Model file for the job. Use its own axes, mm. Face numbers are marked on the shaded views. A direction names the side the tool comes from. Give positions to 0.01 mm unless a question says otherwise; leave off trailing zeros. Loops run counter-clockwise (first coordinate to the right, second up) from the corner with the lowest first, then second, coordinate; pieces in that order, holes last. Notation, with made-up numbers: (12.25, 49.25) -> (61.25, 49.25) arc R31 cw to (61.25, 77.25) -> close; hole circle Ø10 at (31, -14.75). An arc over 180 degrees is marked (long way). Use CSV: the item, a comma, the result in double quotes. Start each with the question number.
(1) Drill centre lines: probe 1 along X at (y, z) = (143.5, 17); probe 2 along X at (y, z) = (-10, 54.5); probe 3 along Z at (x, y) = (19.5, -4). Where is each one in solid material? Low to high.
(2) Cut at A-A on z = -134. Write the cut outline in (x, y).
(3) Cut at D-D on x = 14. Write the cut outline in (y, z).
(4) 3-axis set-ups, long thin cutter, end or side, ignore diameter. For the marked faces 3, 4, 5 and 6: which of +Z, -Z, +X, -X, +Y, -Y reach the whole face in a straight line?
(5) Cut at B-B on x = -82. Write the cut outline in (y, z), then the cut area to 3 significant figures.
(6) Pull direction Y, two halves, no side cores. Call the marked faces 1 and 2: pulls with the +Y half, pulls with the -Y half, needs draft (parallel to the pull), parting line crosses it, or undercut.
(7) Flat gauge pins, fed straight in: pin 1 (5 mm diameter, centred on x = -75, z = -80, fed in from +Y); pin 2 (1 mm diameter, centred on x = 175, y = -15.5, fed in from +Z); pin 3 (10 mm diameter, centred on x = -44.5, z = 64.5, fed in from -Y); pin 4 (7.5 mm diameter, centred on y = -35.27, z = -48.54, fed in from +X). Where does each tip first touch, or does it go through?
(8) Cut at C-C on y = 127. Write the cut outline in (x, z).
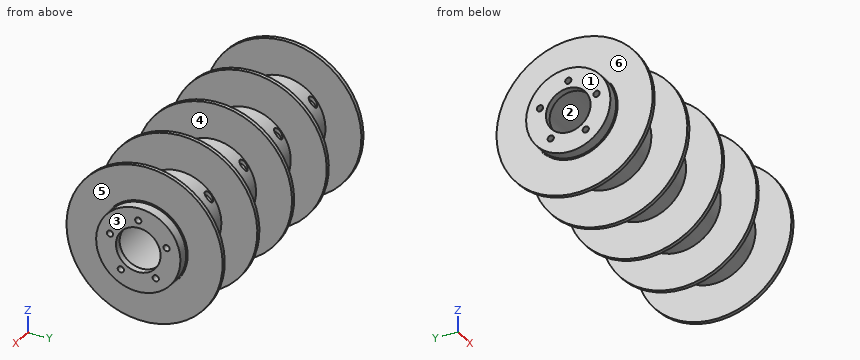
from build123d import *

# Parameters (mm, degrees)
F2_R     = 6.25
F3_DEPTH = 584.001
F4_R     = 7.5
F5_DEPTH = 116


with BuildPart() as f1:
    # F0 (on Front) → F1 (revolve)
    with BuildSketch(Plane.XZ):
        Polygon((4, 157.5), (0, 157.5), (-4, 157.5), (-4, 85), (-128, 85), (-128, 157.5), (-136, 157.5), (-136, 85), (-260, 85), (-260, 157.5), (-268, 157.5), (-268, 87), (-270, 87), (-270, 85), (-292, 85), (-292, 45), (-278, 45), (-278, 79), (0, 79), (278, 79), (278, 45), (292, 45), (292, 85), (270, 85), (270, 87), (268, 87), (268, 157.5), (260, 157.5), (260, 85), (136, 85), (136, 157.5), (128, 157.5), (128, 85), (4, 85), align=None)
    revolve(axis=Axis((-161.670029, 0, 0), (-1, 0, 0)))

    # F2 (on face) → F3 (cut, through all)
    with BuildSketch(Plane.YZ.offset(292)):
        with Locations((0, 60)):
            Circle(F2_R)
        with Locations((-57.063391, 18.54102)):
            Circle(F2_R)
        with Locations((-35.267115, -48.54102)):
            Circle(F2_R)
        with Locations((35.267115, -48.54102)):
            Circle(F2_R)
        with Locations((57.063391, 18.54102)):
            Circle(F2_R)
    extrude(amount=-F3_DEPTH, mode=Mode.SUBTRACT)

    # F4 (on Top) → F5 (cut)
    with BuildSketch(Plane.XY):
        with Locations((-250, 65)):
            Circle(F4_R)
        with Locations((-118, 65)):
            Circle(F4_R)
        with Locations((14, 65)):
            Circle(F4_R)
        with Locations((146, 65)):
            Circle(F4_R)
    extrude(amount=F5_DEPTH, mode=Mode.SUBTRACT)


solid = f1.part
Check result:
1,probe 1,"-268 to -260, -136 to -128, -4 to 4, 128 to 136, 260 to 268"
1,probe 2,"-292 to -278, 278 to 292"
1,probe 3,"-84.91 to -78.9, 78.9 to 84.91"
2,outline,"(-268, -82.77) -> (-260, -82.77) -> (-260, 82.77) -> (-268, 82.77) -> close; (-136, -82.77) -> (-128, -82.77) -> (-128, 82.77) -> (-136, 82.77) -> close; (-4, -82.77) -> (4, -82.77) -> (4, 82.77) -> (-4, 82.77) -> close; (128, -82.77) -> (136, -82.77) -> (136, 82.77) -> (128, 82.77) -> close; (260, -82.77) -> (268, -82.77) -> (268, 82.77) -> (260, 82.77) -> close"
3,outline,"(57.5, 54.17) -> (57.5, 62.6) arc R85 ccw (long way) to (72.5, 44.37) -> (72.5, 31.38) arc R79 cw (long way) to start"
4,face 3,"+Z, -Z, +X, +Y, -Y"
4,face 4,"none"
4,face 5,"+X"
4,face 6,"-X"
5,outline,"circle Ø170 at (0, 0); hole circle Ø158 at (0, 0)"
5,area,"3,090 mm²"
6,face 1,"needs draft"
6,face 2,"undercut"
7,pin 1,"y = 34.91"
7,pin 2,"z = 83.67"
7,pin 3,"y = -60.7"
7,pin 4,"through"
8,outline,"(-268, -93.15) -> (-260, -93.15) -> (-260, 93.15) -> (-268, 93.15) -> close; (-136, -93.15) -> (-128, -93.15) -> (-128, 93.15) -> (-136, 93.15) -> close; (-4, -93.15) -> (4, -93.15) -> (4, 93.15) -> (-4, 93.15) -> close; (128, -93.15) -> (136, -93.15) -> (136, 93.15) -> (128, 93.15) -> close; (260, -93.15) -> (268, -93.15) -> (268, 93.15) -> (260, 93.15) -> close"
